from build123d import *

# Parameters (mm, degrees)
F0_W     = 10
F0_H     = 30
F0_W_2   = 8
F0_H_2   = 15
F0_R     = 17.5
F1_DEPTH = 25


# Not quite as in the source:
# - a feature of the source that left no trace in its solid (it failed there, or was rolled back) is left out


with BuildPart() as f1:
    # F0 (on Top) → F1 (new body)
    with BuildSketch(Plane.XY):
        with Locations((-62.4986458628, -23.6081185268)):
            Rectangle(F0_W, F0_H)
        with Locations((-43.4986458628, -16.1081185268)):
            Rectangle(F0_W_2, F0_H_2)
        Polygon((87.5013541372, 16.3918814732), (-67.4986458628, 16.3918814732), (-67.4986458628, -8.6081185268), (-57.4986458628, -8.6081185268), (-47.4986458628, -8.6081185268), (-39.4986458628, -8.6081185268), (-29.4986458628, -8.6081185268), (-15.4986458628, -8.6081185268), (87.5013541372, -8.6081185268), align=None)
        Polygon((-22.4986458628, -23.6081185268), (-15.4986458628, -8.6081185268), (-29.4986458628, -8.6081185268), align=None)
        with BuildLine():
            ThreePointArc((87.5013541372, -8.6081185268), (155.1930962138, 3.8918814732), (87.5013541372, 16.3918814732))
            Line((87.5013541372, 16.3918814732), (87.5013541372, -8.6081185268))
        make_face()
        with Locations((120.1930962138, 3.8918814732)):
            Circle(F0_R, mode=Mode.SUBTRACT)
    extrude(amount=F1_DEPTH)


solid = f1.part
Can you work these out from the model? Positions are in its coordinate system, mm. A direction names the side the tool comes from. Give positions to 0.01 mm unless a question says otherwise; leave off trailing zeros. Order: outer loops, then holes, each group sorted by start corner. A loop starts at its lowest first (then second) coordinate and runs counter-clockwise, first axis right, second up. Notation, with made-up numbers: (41.25, 77.5) - (68.25, 77.5) arc R33 ccw to (68.25, 106.5) - close; hole circle Ø9 at (30.5, 31.5). An arc over 180 degrees is marked (long way). Write each question's results on one line, items separated by ' | '.
1) On a 3-axis mill with a long thin cutter (end or side, diameter ignored), from which of +Z, -Z, +X, -X, +Y, -Y can I reach the whole of each face in a straight line? I mean faces 4 (the face through (-44, -23.608, 12)), 5 (the face through (11, 16.392, 12)), 6 (the face through (67, 1, 0)). Say none if no direction works.
Final values:
face 4: +Z, -Z, -Y | face 5: +Z, -Z, -X, +Y | face 6: -Z, +X, -X, +Y, -Y
2) Suppose I cut it at B-B, the plane y = 19. Write out the boundary of the cut face in (x, z), then the cut area to 3 significant figures.
Final values:
outline: (88.62, 0) - (111.36, 0) - (111.36, 25) - (88.62, 25) - close; (129.02, 0) - (151.76, 0) - (151.76, 25) - (129.02, 25) - close | area: 1,140 mm^2
3) Suppose I cut it at D-D, the plane x = 74.5. Write out the boundary of the cut face in (y, z).
Final values:
outline: (-8.61, 0) - (16.39, 0) - (16.39, 25) - (-8.61, 25) - close
4) Please list where these lines run through material, in increasing order: line 1 along Y through (x, z) = (120, 14.25); line 2 along X through (y, z) = (-15, 8.5); line 3 along X through (y, z) = (-19.5, 6.5). Write a range as [from, to].
Final values:
line 1: y = [-31.11, -13.61], [21.39, 38.89] | line 2: x = [-67.5, -57.5], [-47.5, -39.5], [-26.52, -18.48], [90.73, 149.66] | line 3: x = [-67.5, -57.5], [-47.5, -39.5], [-24.42, -20.58], [94.16, 146.23]
5) If we mould it in two halves opening along X, with no side actions, what happens to faces 1 (the face through (-67.499, -11, 12)), 2 (the face through (-63, -38.608, 12)), 3 (the face through (155.167, 2.532, 12.325))? For each: pulls with the +X half, pulls with the -X half, needs draft (parallel to the pull), parting line crosses it, or undercut.
Final values:
face 1: pulls with the -X half | face 2: needs draft | face 3: undercut
6) Suppose I cut it at A-A, the plane x = 112.5. Write out the boundary of the cut face in (y, z), then the cut area to 3 significant figures.
Final values:
outline: (-30.25, 0) - (-11.83, 0) - (-11.83, 25) - (-30.25, 25) - close; (19.61, 0) - (38.04, 0) - (38.04, 25) - (19.61, 25) - close | area: 921 mm^2
7) I'm going to push flat-ended pins straight in: pin 1 Ø12.5 at (x, z) = (41.5, 16.5) entering from -Y; pin 2 Ø8 at (x, z) = (114.5, 9.5) entering from -Y; pin 3 Ø3 at (x, z) = (-44.5, 14) entering from -Y; pin 4 Ø2 at (x, y) = (-22, -13.5) entering from -Z. Where does each tip first touch, or does it pass through?
Final values:
pin 1: stops at y = -8.61 | pin 2: stops at y = -31.07 | pin 3: stops at y = -23.61 | pin 4: stops at z = 0
8) Suppose I cut it at C-C, the plane z = 19.5. Write out the boundary of the cut face in (x, y), then the cut area to 3 significant figures.
Final values:
outline: (-67.5, -38.61) - (-57.5, -38.61) - (-57.5, -8.61) - (-47.5, -8.61) - (-47.5, -23.61) - (-39.5, -23.61) - (-39.5, -8.61) - (-29.5, -8.61) - (-22.5, -23.61) - (-15.5, -8.61) - (87.5, -8.61) arc R35 ccw (long way) to (87.5, 16.39) - (-67.5, 16.39) - close; hole circle Ø35 at (120.19, 3.89) | area: 7,250 mm^2
